from build123d import *
from build123d.topology import SkipClean

# Parameters (mm, degrees)
SKETCH5_W           = 50
SKETCH5_H           = 130
BOSS_EXTRUDE1_DEPTH = 150
CUT_EXTRUDE1_START  = -25
CUT_EXTRUDE1_DEPTH  = 15
BOSS_EXTRUDE3_START = 30
SKETCH17_W          = 30
SKETCH17_H          = 40
BOSS_EXTRUDE3_DEPTH = 5
SKETCH10_R          = 8.75
CUT_EXTRUDE3_DEPTH  = 100
SKETCH18_W          = 48.5
SKETCH18_H          = 10
BOSS_EXTRUDE4_DEPTH = 10
BOSS_EXTRUDE5_START = 40
SKETCH18_2_W        = 48.5
SKETCH18_2_H        = 10
BOSS_EXTRUDE5_DEPTH = 10
CHAMFER1_SIZE       = 25
CUT_EXTRUDE5_DEPTH  = 70
FILLET1_DEPTH       = 10
FILLET1_START       = 40
FILLET1_2_DEPTH     = 10
CUT_EXTRUDE6_DEPTH  = 70
FILLET2_R           = 10
BOSS_EXTRUDE6_START = 20
BOSS_EXTRUDE6_DEPTH = 20
FILLET4_R           = 3


with BuildPart() as part:
    # Sketch5 → Boss-Extrude1 (new body)
    with BuildSketch(Plane(origin=(0, 0, 0), x_dir=(1, 0, 0), z_dir=(0, 1, 0))):
        with Locations((25, 65)):
            Rectangle(SKETCH5_W, SKETCH5_H)
    extrude(amount=BOSS_EXTRUDE1_DEPTH)

    # Sketch7 → Cut-Extrude1 (cut, symmetric)
    with BuildSketch(Plane(origin=(50, 0, 0), x_dir=(0, 0, -1), z_dir=(1, 0, 0)).offset(CUT_EXTRUDE1_START)):
        Polygon((130, 0), (130, 133.702332435), (0, 42.675352467), (0, 0), align=None)
        Polygon((0, 50), (130, 141.026979967), (130, 150), (0, 150), align=None)
    extrude(amount=CUT_EXTRUDE1_DEPTH, both=True, mode=Mode.SUBTRACT)

    # Sketch17 → Boss-Extrude3 (add)
    with BuildSketch(Plane(origin=(0, 275.412054826, -321.921776796), x_dir=(1, 0, 0), z_dir=(0, -0.819152044288993, -0.5735764363510444)).offset(BOSS_EXTRUDE3_START)):
        with Locations((25, 354.293228142)):
            Rectangle(SKETCH17_W, SKETCH17_H)
    extrude(amount=-BOSS_EXTRUDE3_DEPTH)

    # Sketch10 → Cut-Extrude3 (cut)
    with BuildSketch(Plane(origin=(0, 33.550503583, 23.49231552), x_dir=(1, 0, 0), z_dir=(0, 0.819152044288993, 0.5735764363510444))):
        with Locations(Location((25, 68.178273127, 0), (0, 0, 90))):
            Circle(SKETCH10_R)
    extrude(amount=-CUT_EXTRUDE3_DEPTH, mode=Mode.SUBTRACT)

    # Sketch18 → Boss-Extrude4 (add)
    with BuildSketch(Plane(origin=(0, 0, 0), x_dir=(0, 0, -1), z_dir=(1, 0, 0))):
        with Locations((24.25, 155)):
            Rectangle(SKETCH18_W, SKETCH18_H)
    extrude(amount=BOSS_EXTRUDE4_DEPTH)

    # Sketch18<2> → Boss-Extrude5 (add)
    with BuildSketch(Plane(origin=(0, 0, 0), x_dir=(0, 0, -1), z_dir=(1, 0, 0)).offset(BOSS_EXTRUDE5_START)):
        with Locations((24.25, 155)):
            Rectangle(SKETCH18_2_W, SKETCH18_2_H)
    extrude(amount=BOSS_EXTRUDE5_DEPTH)

    # Chamfer1
    chamfer1_edges = [part.edges().sort_by_distance(p)[0] for p in [
        (5, 160, 0),
        (45, 160, 0),
    ]]
    chamfer(chamfer1_edges, length=CHAMFER1_SIZE)

    # Sketch21 → Cut-Extrude5 (cut)
    with BuildSketch(Plane(origin=(0, 0, 0), x_dir=(0, 0, -1), z_dir=(1, 0, 0))):
        Polygon((62.42420648, 63.190535225), (51.526254189, 78.754424066), (18.760172418, 55.811366612), (29.658124708, 40.247477771), align=None)
        Polygon((69.307123716, 53.360710693), (36.541041945, 30.417653239), (32.52600689, 36.151717549), (65.292088662, 59.094775003), align=None)
    extrude(amount=CUT_EXTRUDE5_DEPTH, mode=Mode.SUBTRACT)

    # Fillet1: read off the stored shape, not the designer's step
    # Fillet1 outline → Fillet1 (add)
    with BuildSketch(Plane.YZ):
        with BuildLine():
            Line((30.417653239, -36.541041945), (33.285535421, -40.636802166))
            ThreePointArc((33.285535421, -40.636802166), (32.457256878, -36.900679096), (34.513413461, -33.673159763))
            Line((34.513413461, -33.673159763), (30.417653239, -36.541041945))
        make_face()
        with BuildLine():
            ThreePointArc((43.115359953, -33.75388493), (42.287081409, -30.01776186), (44.343237992, -26.790242527))
            Line((44.343237992, -26.790242527), (40.247477771, -29.658124708))
            Line((40.247477771, -29.658124708), (43.115359953, -33.75388493))
        make_face()
    extrude(amount=FILLET1_DEPTH)

    # Fillet1 2 outline → Fillet1 2 (add)
    with BuildSketch(Plane.YZ.offset(FILLET1_START)):
        with BuildLine():
            Line((30.417653239, -36.541041945), (33.285535421, -40.636802166))
            ThreePointArc((33.285535421, -40.636802166), (32.457256878, -36.900679096), (34.513413461, -33.673159763))
            Line((34.513413461, -33.673159763), (30.417653239, -36.541041945))
        make_face()
        with BuildLine():
            ThreePointArc((43.115359953, -33.75388493), (42.287081409, -30.01776186), (44.343237992, -26.790242527))
            Line((44.343237992, -26.790242527), (40.247477771, -29.658124708))
            Line((40.247477771, -29.658124708), (43.115359953, -33.75388493))
        make_face()
    extrude(amount=FILLET1_2_DEPTH)

    # Sketch22 → Cut-Extrude6 (cut)
    with BuildSketch(Plane.ZY):
        Polygon((-115, 0), (-95, 20), (-65, 0), align=None)
    extrude(amount=-CUT_EXTRUDE6_DEPTH, mode=Mode.SUBTRACT)

    # Fillet2
    fillet2_edges = [part.edges().sort_by_distance(p)[0] for p in [
        (25, 50, 0),
    ]]
    fillet(fillet2_edges, radius=FILLET2_R)

    # Sketch23 → Boss-Extrude6 (add)
    with SkipClean():  # the faces are left unmerged after this step: merging them gives an invalid solid
        with BuildSketch(Plane(origin=(0, 33.550503583, 23.49231552), x_dir=(1, 0, 0), z_dir=(0, 0.819152044288993, 0.5735764363510445)).offset(BOSS_EXTRUDE6_START)):
            with BuildLine():
                Line((40, 69.739442097), (32.180703308, 63.178273127))
                ThreePointArc((32.180703308, 63.178273127), (31.983337112, 62.906129088), (31.77566264, 62.64176739))
                ThreePointArc((31.77566264, 62.64176739), (32.241088602, 60.832062958), (34.109066137, 60.880139798))
                Line((34.109066137, 60.880139798), (40, 65.823220229))
                Line((40, 65.823220229), (40, 69.739442097))
            make_face()
            with BuildLine():
                ThreePointArc((18.22433736, 62.64176739), (18.016662888, 62.906129088), (17.819296692, 63.178273127))
                Line((17.819296692, 63.178273127), (10, 69.739442097))
                Line((10, 69.739442097), (10, 65.823220229))
                Line((10, 65.823220229), (15.890933863, 60.880139798))
                ThreePointArc((15.890933863, 60.880139798), (17.758911398, 60.832062958), (18.22433736, 62.64176739))
            make_face()
        extrude(amount=-BOSS_EXTRUDE6_DEPTH)

    # Fillet4
    fillet4_edges = [part.edges().sort_by_distance(p)[0] for p in [
        (40, 79.496672114, -24.691145529),
        (10, 79.496672114, -24.691145529),
    ]]
    fillet(fillet4_edges, radius=FILLET4_R)


solid = part.part
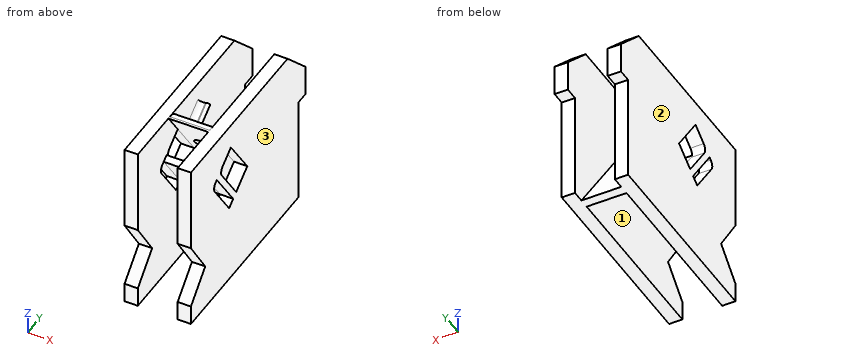
Source: CAD feature listing. Evaluate the final solid. Frame: model axes, mm. Face numbers are marked on the shaded views. Round coordinates to 2 decimals unless told otherwise and drop trailing zeros. Order: outer loops, then holes, each group sorted by start corner. A loop starts at its lowest first (then second) coordinate and runs counter-clockwise, first axis right, second up. Notation, with made-up numbers: (19.5, 88.5) - (55.5, 88.5) arc R35 cw to (55.5, 127.5) - close; hole circle Ø1 at (41.25, -17). An arc over 180 degrees is marked (long way). Use a Markdown table: item, result. Add a question column.
1. Section query C-C (z = -67). Return the cut outline in (x, y), then the cut area to 3 significant figures.
2. Section query D-D (y = 38). Return the cut outline in (x, z), then the cut area to 3 significant figures.
3. Line query: probe 1 along X at (y, z) = (34, -74.5); probe 2 along Y at (x, z) = (46.5, -49); probe 3 along Y at (x, z) = (22, -55.5). Output: solid intervals per line, ascending.
4. Section query A-A (y = 13). Return the cut outline in (x, z).
5. First-contact query: pin 1 (5 mm diameter, centred on x = 19, z = -97, fed in from +Y); pin 2 (3 mm diameter, centred on x = 4, y = 153.5, fed in from -Z); pin 3 (3 mm diameter, centred on x = 18, y = 126.5, fed in from +Z). Flat tips, straight axial feed; report the tip coordinate or a pass-through.
6. Section query B-B (x = 45.5). Return the cut outline in (y, z), then the cut area to 3 significant figures.
7. Mould query, pull axis X, two halves, no side actions, for the marked faces 1, 2 and 3. Classes: +X half, -X half, draft (parallel to the pull), parting line (faces both ways), or undercut.
Derived:
| question | item | result |
|---|---|---|
| 1 | outline | (0, 1.33) - (10, 1.33) - (10, 51.75) - (0, 51.75) - close; (0, 56.66) - (10, 56.66) - (10, 89.59) - (40, 89.59) - (40, 56.66) - (50, 56.66) - (50, 150) - (40, 150) - (40, 96.91) - (10, 96.91) - (10, 150) - (0, 150) - close; (40, 1.33) - (50, 1.33) - (50, 51.75) - (40, 51.75) - close |
| 1 | area | 3,090 mm2 |
| 2 | outline | (0, -130) - (10, -130) - (10, -47.37) - (0, -47.37) - close; (0, -35.17) - (50, -35.17) - (50, 0) - (40, 0) - (40, -31.23) - (10, -31.23) - (10, 0) - (0, 0) - close; (40, -130) - (50, -130) - (50, -47.37) - (40, -47.37) - close |
| 2 | area | 2,470 mm2 |
| 3 | probe 1 | 0 to 10, 40 to 50 |
| 3 | probe 2 | 0 to 39.14, 47.69 to 53.79, 76.99 to 150 |
| 3 | probe 3 | 53.93 to 58.34, 81.54 to 88.86 |
| 4 | outline | (0, -130) - (10, -130) - (10, -102) - (0, -102) - close; (0, -84.5) - (10, -84.5) - (10, 0) - (0, 0) - close; (40, -130) - (50, -130) - (50, -102) - (40, -102) - close; (40, -84.5) - (50, -84.5) - (50, 0) - (40, 0) - close |
| 5 | pin 1 | y = 119.67 |
| 5 | pin 2 | z = -48.5 |
| 5 | pin 3 | z = -107.11 |
| 6 | outline | (0, -130) - (150, -130) - (150, -48.5) - (160, -48.5) - (160, -25) - (135, 0) - (0, 0) - (0, -65) - (20, -95) - (0, -115) - close; hole (33.29, -40.64) - (53.36, -69.31) - (59.09, -65.29) - (36.15, -32.53) - (34.51, -33.67) arc R5 ccw to start; hole (43.12, -33.75) - (63.19, -62.42) - (78.75, -51.53) - (55.81, -18.76) - (44.34, -26.79) arc R5 ccw to start |
| 6 | area | 18,100 mm2 |
| 7 | face 1 | undercut |
| 7 | face 2 | -X half |
| 7 | face 3 | +X half |
